from build123d import *

# Parameters (mm, degrees)
BOSS_EXTRUDE1_DEPTH = 26
SKETCH2_R           = 2.5
CUT_EXTRUDE1_DEPTH  = 46
CUT_EXTRUDE2_DEPTH  = 396
FILLET1_R           = 3
FILLET2_R           = 5


with BuildPart() as part:
    # Sketch1 → Boss-Extrude1 (new body)
    with BuildSketch(Plane.XY):
        Polygon((0, 0), (0, 395), (-45, 395), (-45, 391), (-4, 391), (-4, 0), align=None)
    extrude(amount=BOSS_EXTRUDE1_DEPTH)

    # Sketch2 → Cut-Extrude1 (cut, through all)
    with BuildSketch(Plane(origin=(0, 0, 0), x_dir=(0, 0, -1), z_dir=(1, 0, 0))):
        with Locations((-13, 195)):
            Circle(SKETCH2_R)
        with Locations((-13, 115)):
            Circle(SKETCH2_R)
        with Locations((-13, 35)):
            Circle(SKETCH2_R)
        with Locations((-13, 275)):
            Circle(SKETCH2_R)
        with Locations((-13, 355)):
            Circle(SKETCH2_R)
    extrude(amount=-CUT_EXTRUDE1_DEPTH, mode=Mode.SUBTRACT)

    # Sketch3 → Cut-Extrude2 (cut, through all)
    with BuildSketch(Plane(origin=(0, 395, 0), x_dir=(1, 0, 0), z_dir=(0, 1, 0))):
        with BuildLine():
            Line((-30, -6.5), (-17, -6.5))
            ThreePointArc((-17, -6.5), (-10.5, -13), (-17, -19.5))
            Line((-17, -19.5), (-30, -19.5))
            ThreePointArc((-30, -19.5), (-36.5, -13), (-30, -6.5))
        make_face()
    extrude(amount=-CUT_EXTRUDE2_DEPTH, mode=Mode.SUBTRACT)

    # Fillet1
    fillet1_edges = [part.edges().sort_by_distance(p)[0] for p in [
        (-4, 391, 13),
    ]]
    fillet(fillet1_edges, radius=FILLET1_R)

    # Fillet2
    fillet2_edges = [part.edges().sort_by_distance(p)[0] for p in [
        (0, 395, 13),
    ]]
    fillet(fillet2_edges, radius=FILLET2_R)


solid = part.part
Read the model definition and answer for the solid it produces. Units are mm, in the model's axes. A direction names the side the tool comes from. Coordinates: 2 decimals unless noted, no trailing zeros. Write each loop counter-clockwise with the first axis right and the second up, starting at its lowest first coordinate (ties: lowest second). Pieces come first, ordered by that corner, then holes. Notation, with made-up numbers: (8, -1.75) -> (18, -1.75) arc R24 cw to (18, 14.25) -> close; hole circle Ø1 at (31, 60.25). An arc over 180 degrees is marked (long way). Return JSON: item names as keys, results as strings.
(1) The part is cut by section B-B on y = 238. Give the vertices of the cut face in (x, z), then the cut area to 3 significant figures.
Answers below:
{"outline": "(-4, 0) -> (0, 0) -> (0, 26) -> (-4, 26) -> close", "area": "104 mm^2"}
(2) For a pull along Z with two mould halves and no side action, classify faces 4 (the flat face through (-26, 391, 21)), 5 (the cylindrical face through (-36.5, 393, 13.1)), 6 (the flat face through (-1, 198, 26)) as pulls with the +Z half, pulls with the -Z half, needs draft (parallel to the pull), parting line crosses it, or undercut.
Answers below:
{"face 4": "needs draft", "face 5": "undercut", "face 6": "pulls with the +Z half"}
(3) Which of the six approach directions +Z, -Z, +X, -X, +Y, -Y give full straight-line access (tool end or side, diameter ignored) to faces 1 (the cylindrical face through (-10.5, 393, 12.9)), 2 (the flat face through (-4, 197, 10)), 3 (the flat face through (-25, 395, 21))?
Answers below:
{"face 1": "+Y, -Y", "face 2": "+Z, -Z, -X, -Y", "face 3": "+Z, -Z, +X, -X, +Y"}
(4) Each of these flat-tipped pins is pushed along its axis until it touches: P1, Ø10, axis at x = -10, z = 12.5, coming from the -Y side; P2, Ø6.5, axis at y = 275, z = 13, coming from the -X side; P3, Ø2, axis at x = -7.5, z = 16.5, coming from the -Y side. Where does it stop, or does it pass through?
Answers below:
{"P1": "y = 390.24", "P2": "x = -4", "P3": "y = 390.96"}
(5) The part is cut by section A-A on x = -26.5. Give the vertices of the cut face in (y, z), then the cut area to 3 significant figures.
Answers below:
{"outline": "(391, 0) -> (395, 0) -> (395, 6.5) -> (391, 6.5) -> close; (391, 19.5) -> (395, 19.5) -> (395, 26) -> (391, 26) -> close", "area": "52.0 mm^2"}
(6) Consider line 1 along Z through (x, y) = (-1.55, 195); line 2 along Y through (x, z) = (-1.55, 13); line 3 along Y through (x, z) = (-1.65, 13). Determine where each line is inside the solid, lowest interval first. Write a range as from..to.
Answers below:
{"line 1": "0..10.5, 15.5..26", "line 2": "0..32.5, 37.5..112.5, 117.5..192.5, 197.5..272.5, 277.5..352.5, 357.5..393.62", "line 3": "0..32.5, 37.5..112.5, 117.5..192.5, 197.5..272.5, 277.5..352.5, 357.5..393.71"}
(7) The part is cut by section C-C on x = -41.5. Give the vertices of the cut face in (y, z), then the cut area to 3 significant figures.
Answers below:
{"outline": "(391, 0) -> (395, 0) -> (395, 26) -> (391, 26) -> close", "area": "104 mm^2"}
